Autodesk Inventor part; units mm, degrees
ref_plane "YZ Plane" through (0, 0, 0) normal (1, 0, 0) x (0, 1, 0)
ref_plane "XZ Plane" through (0, 0, 0) normal (0, 1, 0) x (-1, 0, 0)
ref_plane "XY Plane" through (0, 0, 0) normal (0, 0, 1) x (1, 0, 0)
sketch "Sketch1" plane through (0, 0, 0) normal (0, 1, 0) x (-1, 0, 0)
  circle A0 centre (0, 0) radius 50
  dimension "d0" = 100
extrude "Extrusion1" add sketch "Sketch1" along normal blind 7
sketch "Sketch2" plane through (0, 7, 0) normal (0, 1, 0) x (1, 0, 0)
  line L0 (0, 0) -> (50, 0)
  line L1 (50, 0) -> (50, 3)
  line L2 (50, 3) -> (0, 3)
  line L3 (0, 3) -> (0, 0)
  dimension "d3" = 50
  dimension "d4" = 3
extrude "Extrusion2" add sketch "Sketch2" along normal blind 20
sketch "Sketch3" plane through (0, 7, 0) normal (0, 1, 0) x (1, 0, 0)
  line L0 (0, 3) -> (0, 0)
  line L1 (0, 0) -> (3, 0)
  line L2 (3, 0) -> (3, 50)
  line L3 (3, 50) -> (0, 50)
  line L4 (0, 50) -> (0, 0)
  dimension "d7" = 3
  dimension "d8" = 50
extrude "Extrusion3" add sketch "Sketch3" along normal blind 20
sketch "Sketch4" plane through (0, 7, 0) normal (0, 1, 0) x (1, 0, 0)
  line L0 (0, 0) -> (0, 50)
  line L1 (0, 50) -> (-50, 50)
  line L2 (-50, 50) -> (-50, -50)
  line L3 (-50, -50) -> (0, -50)
  line L4 (0, -50) -> (0, 50)
  line L5 (50, 0) -> (0, 0)
  line L6 (0, 0) -> (50, 0)
  line L7 (50, 0) -> (50, -50)
  line L8 (50, -50) -> (0, -50)
  line L9 (0, -50) -> (0, 0)
  dimension "d11" = 50
  dimension "d12" = 100
  dimension "d13" = 50
  dimension "d14" = 50
extrude "Extrusion4" cut sketch "Sketch4" against normal blind 7
sketch "Sketch5" plane through (0, 7, 0) normal (0, 1, 0) x (1, 0, 0)
  line L0 (3, 49.9099) -> (3, 3)
  line L1 (3, 3) -> (49.9099, 3)
  point P0 (0, 0)
  point P1 (23, 13)
  dimension "d24" = 20
  dimension "d25" = 10
hole "Hole1" at (23, 7, -13) direction (0, -1, 0) diameter 6.5 end through all counterbore diameter 10.5 counterbore depth 5
fillet "Fillet1" radius 20 1 edges at (1.5, 27, -50)
fillet "Fillet2" radius 20 1 edges at (50, 27, -1.5)
properties part number "euro_box_corner_r"
CAD build for the part. Positions are in the model's coordinates, mm. A direction names the side the tool comes from. Coordinates: 2 decimals unless noted, no trailing zeros. Order: outer loops, then holes, each group sorted by start corner. A loop starts at its lowest first (then second) coordinate and runs counter-clockwise, first axis right, second up. Notation, with made-up numbers: (74.25, 80.5) -> (111.25, 80.5) arc R12 ccw to (111.25, 97.5) -> close; hole circle Ø11 at (73, 84.25). An arc over 180 degrees is marked (long way). Use one line per item in the form item = value. Start each with the question number.
1) Drop flat-ended pins along their axis: pin 1 (6 mm diameter, centred on x = 31.5, y = 13, fed in from -Z); pin 2 (8 mm diameter, centred on y = 21, z = -44.5, fed in from +X); pin 3 (11.5 mm diameter, centred on x = 25.5, z = -10.5, fed in from +Y). Give the stop position or say it passes through.
2) Band-saw the part on C-C on y = 3.5. Give the cut face in (x, z).
3) Tool access for faces 4 (the cylindrical face through (26.19, 4.46, -17.17)), 5 (the flat face through (22, 7, -21)), 6 (the cylindrical face through (24.978, 0.986, -15.579)): list every direction of +Z, -Z, +X, -X, +Y, -Y with a clear straight run to the whole face (end or side of a thin tool).
4) Band-saw the part on A-A on x = 23. Give the cut face in (y, z).
5) Band-saw the part on B-B on z = -13. Give the cut face in (x, y).
6) Drill centre lines: L1, parallel to X at y = 21, z = -8; L2, parallel to Z at x = 43, y = 21.5; L3, parallel to Y at x = 36, z = -14. Where is each one in solid material? Low to high. Write a range as [from, to].
7) Band-saw the part on D-D on x = 45. Give the cut face in (y, z), then the cut area to 3 significant figures.
8) Pull direction X, two halves, no side cores. Call faces 1 (the flat face through (0, 13, -25)), 2 (the flat face through (26.4, 2, -13.1)), 3 (the cylindrical face through (43.986, 21.297, -1.521)): +X half, -X half, draft (parallel to the pull), parting line (faces both ways), or undercut.
Entries:
q1.pin_1 = -3
q1.pin_2 = 3
q1.pin_3 = 7
q2.outline = (0, -50) arc R50 ccw to (50, 0) -> (0, 0) -> close; hole circle Ø10.5 at (23, -13)
q3.face_4 = +Y
q3.face_5 = -Z, +X, +Y
q3.face_6 = +Y, -Y
q4.outline = (0, -44.4) -> (7, -44.4) -> (7, -18.25) -> (2, -18.25) -> (2, -16.25) -> (0, -16.25) -> close; (0, -9.75) -> (2, -9.75) -> (2, -7.75) -> (7, -7.75) -> (7, -3) -> (27, -3) -> (27, 0) -> (0, 0) -> close
q5.outline = (0, 0) -> (19.75, 0) -> (19.75, 2) -> (17.75, 2) -> (17.75, 7) -> (3, 7) -> (3, 27) -> (0, 27) -> close; (26.25, 0) -> (48.28, 0) -> (48.28, 7) -> (28.25, 7) -> (28.25, 2) -> (26.25, 2) -> close
q6.L1 = [0, 3]
q6.L2 = [-3, 0]
q6.L3 = [0, 7]
q7.outline = (0, -21.79) -> (7, -21.79) -> (7, -3) -> (20.23, -3) -> (20.23, 0) -> (0, 0) -> close
q7.area = 192 mm2
q8.face_1 = -X half
q8.face_2 = undercut
q8.face_3 = +X half
